```python
from build123d import *

# Parameters (mm, degrees)
SKETCH_2_R          = 2.1
SKETCH_2_R_2        = 2.6
EXTRUDE_1_DEPTH     = 5
CUT_EXTRUDE_1_DEPTH = 5
SKETCH_5_W          = 46.5
SKETCH_5_H          = 4
CUT_EXTRUDE_2_DEPTH = 5
CHAMFER_2_SIZE      = 3


with BuildPart() as part:
    # 草图2 → 凸台-拉伸1 (new body)
    with BuildSketch(Plane.XY):
        with BuildLine():
            Line((-23.25, 0), (23.25, 0))
            Line((23.25, 0), (23.25, -16))
            Line((23.25, -16), (37.25, -16))
            Line((37.25, -16), (37.25, 8))
            Line((37.25, 8), (72.368161114, 47.692911962))
            ThreePointArc((72.368161114, 47.692911962), (73.426469111, 54.669637405), (67.5, 58.5))
            Line((67.5, 58.5), (55.5, 58.5))
            Line((55.5, 58.5), (37.5, 65))
            Line((37.5, 65), (-37.5, 65))
            Line((-37.5, 65), (-55.5, 58.5))
            Line((-55.5, 58.5), (-67.5, 58.5))
            ThreePointArc((-67.5, 58.5), (-73.426469111, 54.669637405), (-72.368161114, 47.692911962))
            Line((-72.368161114, 47.692911962), (-37.25, 8))
            Line((-37.25, 8), (-37.25, -16))
            Line((-37.25, -16), (-23.25, -16))
            Line((-23.25, -16), (-23.25, 0))
        make_face()
        with Locations((28, -9)):
            Circle(SKETCH_2_R, mode=Mode.SUBTRACT)
        with Locations((28, 3)):
            Circle(SKETCH_2_R, mode=Mode.SUBTRACT)
        with Locations((44.307987485, 25.786824772)):
            Circle(SKETCH_2_R_2, mode=Mode.SUBTRACT)
        with Locations((56.235308207, 39.267886318)):
            Circle(SKETCH_2_R_2, mode=Mode.SUBTRACT)
        with Locations((62.198968568, 46.008417091)):
            Circle(SKETCH_2_R_2, mode=Mode.SUBTRACT)
        with Locations((67.5, 52)):
            Circle(SKETCH_2_R_2, mode=Mode.SUBTRACT)
        with Locations((44, 40)):
            Circle(SKETCH_2_R_2, mode=Mode.SUBTRACT)
        with Locations((44, 52)):
            Circle(SKETCH_2_R_2, mode=Mode.SUBTRACT)
        with Locations((52, 52)):
            Circle(SKETCH_2_R_2, mode=Mode.SUBTRACT)
        with Locations((35, 58)):
            Circle(SKETCH_2_R_2, mode=Mode.SUBTRACT)
        with Locations((-67.5, 52)):
            Circle(SKETCH_2_R_2, mode=Mode.SUBTRACT)
        with Locations((-62.198968568, 46.008417091)):
            Circle(SKETCH_2_R_2, mode=Mode.SUBTRACT)
        with Locations((-56.235308207, 39.267886318)):
            Circle(SKETCH_2_R_2, mode=Mode.SUBTRACT)
        with Locations((-44.307987485, 25.786824772)):
            Circle(SKETCH_2_R_2, mode=Mode.SUBTRACT)
        with Locations((-44, 40)):
            Circle(SKETCH_2_R_2, mode=Mode.SUBTRACT)
        with Locations((-52, 52)):
            Circle(SKETCH_2_R_2, mode=Mode.SUBTRACT)
        with Locations((-44, 52)):
            Circle(SKETCH_2_R_2, mode=Mode.SUBTRACT)
        with Locations((-35, 58)):
            Circle(SKETCH_2_R_2, mode=Mode.SUBTRACT)
        with Locations((-28, -9)):
            Circle(SKETCH_2_R, mode=Mode.SUBTRACT)
        with Locations((-28, 3)):
            Circle(SKETCH_2_R, mode=Mode.SUBTRACT)
    extrude(amount=EXTRUDE_1_DEPTH)

    # 草图3 → 切除-拉伸1 (cut)
    with BuildSketch(Plane.XY.offset(5)):
        Polygon((-26.219338455, 53), (26.219338455, 53), (36, 45.675774443), (36, 19.675774443), (26.492733991, 12), (-26.492733991, 12), (-36, 19.675774443), (-36, 45.675774443), align=None)
    extrude(amount=-CUT_EXTRUDE_1_DEPTH, mode=Mode.SUBTRACT)

    # 草图5 → 切除-拉伸2 (cut)
    with BuildSketch(Plane.XY.offset(5)):
        with Locations((0, 2)):
            Rectangle(SKETCH_5_W, SKETCH_5_H)
    extrude(amount=-CUT_EXTRUDE_2_DEPTH, mode=Mode.SUBTRACT)

    # 倒角2
    chamfer_2_edges = [part.edges().sort_by_distance(p)[0] for p in [
        (-23.25, 4, 2.5),
        (23.25, 4, 2.5),
    ]]
    chamfer(chamfer_2_edges, length=CHAMFER_2_SIZE)


solid = part.part
```
Here's how the part is built. I have some questions about the finished solid (model axes, mm). A direction names the side the tool comes from. Round coordinates to 2 decimals unless told otherwise and drop trailing zeros. Write each loop counter-clockwise with the first axis right and the second up, starting at its lowest first coordinate (ties: lowest second). Pieces come first, ordered by that corner, then holes.
Q1. If we section it at C-C on x = -44: Write out the boundary of the cut face in (y, z).
Q2. If we section it at B-B on y = 17.5: Write out the boundary of the cut face in (x, z).
Q3. If we mould it in two halves opening along X, with no side actions, what happens to faces 6 (the cylindrical face through (42.245, 24.205, 2.465)), 7 (the flat face through (-46.374, 61.796, 2.465)), 8 (the cylindrical face through (73.47, 54.57, 2.46)), 9 (the flat face through (30, -16, 2))? For each: +X half, -X half, draft (parallel to the pull), parting line (faces both ways), or undercut.
Q4. If we section it at A-A on x = 11: Write out the boundary of the cut face in (y, z).
Q5. If we section it at D-D on z = 3.05: Give the number of separate pieces and of enclosed holes in the cut face, plus the area to 3 significant figures.
Q6. Will these pins go through, and if not, where does the flat tip stop? P1, Ø3, axis at y = 41.5, z = 3, coming from the -X side; P2, Ø2, axis at y = 12.5, z = 1.5, coming from the +X side; P3, Ø2, axis at y = 2, z = 0.5, coming from the +X side.
Q7. Which directions (+Z, -Z, +X, -X, +Y, -Y) give clear straight access to the entire face, cutting with the end or side of a thin tool? Please do faces 1 (the flat face through (37.25, -4, 2)), 2 (the flat face through (46.626, 61.704, 2.465)), 3 (the flat face through (-21.73, 2.52, 2.53)), 4 (the flat face through (-30, -16, 2)), 5 (the flat face through (-31.178, 49.287, 2.535)).
Q8. Please list where these lines run through material, in increasing order: probe 1 along Y at (x, z) = (9.5, 4.15); probe 2 along X at (y, z) = (0, 2.2); probe 3 along X at (y, z) = (40.5, 1.1).
Answer below:
1. outline: (15.63, 0) - (23.21, 0) - (23.21, 5) - (15.63, 5) - close; (28.37, 0) - (37.4, 0) - (37.4, 5) - (28.37, 5) - close; (42.6, 0) - (49.4, 0) - (49.4, 5) - (42.6, 5) - close; (54.6, 0) - (62.65, 0) - (62.65, 5) - (54.6, 5) - close
2. outline: (-45.66, 0) - (-33.31, 0) - (-33.31, 5) - (-45.66, 5) - close; (33.31, 0) - (45.66, 0) - (45.66, 5) - (33.31, 5) - close
3. face 6: undercut
3. face 7: -X half
3. face 8: +X half
3. face 9: draft
4. outline: (4, 0) - (12, 0) - (12, 5) - (4, 5) - close; (53, 0) - (65, 0) - (65, 5) - (53, 5) - close
5. separate pieces: 1
5. enclosed holes: 21
5. area: 4,200 mm2
6. P1: stops at x = -68.22
6. P2: stops at x = 42.12
6. P3: stops at x = 37.25
7. face 1: +Z, -Z, +X, -Y
7. face 2: +Z, -Z, +X, +Y
7. face 3: +Z, -Z, -Y
7. face 4: +Z, -Z, +X, -X, -Y
7. face 5: +Z, -Z
8. probe 1: y = 4 to 12, 53 to 65
8. probe 2: x = -37.25 to -23.25, 23.25 to 37.25
8. probe 3: x = -66 to -58.52, -53.95 to -46.55, -41.45 to -36, 36 to 41.45, 46.55 to 53.95, 58.52 to 66
